Could you check a few things on this model? Use its own coordinates, in mm. A direction names the side the tool comes from. Round coordinates to 2 decimals unless told otherwise and drop trailing zeros. Loops run counter-clockwise (first coordinate to the right, second up) from the corner with the lowest first, then second, coordinate; pieces in that order, holes last. Notation, with made-up numbers: (-34.5, -8) - (23.5, -8) arc R22 ccw to (23.5, 28) - close; hole circle Ø1 at (-26.5, -32). An arc over 180 degrees is marked (long way). Answer as CSV lines item,"result". Start each with the question number.
1) Suppose I cut it at B-B, the plane z = 96. Count the separate pieces of the cut face and the enclosed holes in it, then the cut area to 3 significant figures.
2) I'm going to push flat-ended pins straight in: pin 1 Ø3.5 at (y, z) = (0.5, 80.5) entering from +X; pin 2 Ø5 at (x, y) = (16, 1.5) entering from +Z; pin 3 Ø0.5 at (x, z) = (29.5, 173.5) entering from -Y; pin 4 Ø0.5 at (x, z) = (29, 80) entering from +Y. Where does each tip first touch, or does it pass through?
3) Please list where these lines run through material, in increasing order: line 1 along X through (y, z) = (8, 193); line 2 along X through (y, z) = (-1, 208); line 3 along Y through (x, z) = (8, 213).
4) We'd pull the mould along Y, two halves only. Please class faces 5 (the face through (-5, -10, 118)), 6 (the face through (-3.9, 0, 118)), 7 (the face through (23.9, 0, 118)), 8 (the face through (5, 5, 0)): pulls with the +Y half, pulls with the -Y half, needs draft (parallel to the pull), parting line crosses it, or undercut.
5) Suppose I cut it at A-A, the plane x = 10. Write out the boundary of the cut face in (y, z), then the cut area to 3 significant figures.
6) Which directions (+Z, -Z, +X, -X, +Y, -Y) give clear straight access to the entire face, cutting with the end or side of a thin tool? Please do faces 1 (the face through (10, 8.2, 118)), 2 (the face through (20, 3.9, 118)), 3 (the face through (5, 5, 240)), 4 (the face through (0, -3.9, 118)).
```python
from build123d import *

# Parameters (mm, degrees)
SALIENTE_EXTRUIR1_DEPTH = 240


with BuildPart() as part:
    # Croquis1 → Saliente-Extruir1 (new body)
    with BuildSketch(Plane.XY):
        with BuildLine():
            Line((-10, 8.5), (-10, 2.3))
            Line((-10, 2.3), (-8.2, 2.3))
            Line((-8.2, 2.3), (-8.2, 5.5))
            Line((-8.2, 5.5), (-6.348528137, 5.5))
            Line((-6.348528137, 5.5), (-4.485786438, 3.6372583))
            ThreePointArc((-4.485786438, 3.6372583), (-4.052240935, 2.988411603), (-3.9, 2.223044738))
            Line((-3.9, 2.223044738), (-3.9, 0))
            Line((-3.9, 0), (-3.9, -2.223044738))
            ThreePointArc((-3.9, -2.223044738), (-4.052240935, -2.988411603), (-4.485786438, -3.6372583))
            Line((-4.485786438, -3.6372583), (-6.348528137, -5.5))
            Line((-6.348528137, -5.5), (-8.2, -5.5))
            Line((-8.2, -5.5), (-8.2, -2.3))
            Line((-8.2, -2.3), (-10, -2.3))
            Line((-10, -2.3), (-10, -8.5))
            ThreePointArc((-10, -8.5), (-9.560660172, -9.560660172), (-8.5, -10))
            Line((-8.5, -10), (-2.3, -10))
            Line((-2.3, -10), (-2.3, -8.2))
            Line((-2.3, -8.2), (-5.5, -8.2))
            Line((-5.5, -8.2), (-5.5, -6.348528137))
            Line((-5.5, -6.348528137), (-3.6372583, -4.485786438))
            ThreePointArc((-3.6372583, -4.485786438), (-2.988411603, -4.052240935), (-2.223044738, -3.9))
            Line((-2.223044738, -3.9), (0, -3.9))
            Line((0, -3.9), (2.223044738, -3.9))
            ThreePointArc((2.223044738, -3.9), (2.988411603, -4.052240935), (3.6372583, -4.485786438))
            Line((3.6372583, -4.485786438), (5.5, -6.348528137))
            Line((5.5, -6.348528137), (5.5, -8.2))
            Line((5.5, -8.2), (2.3, -8.2))
            Line((2.3, -8.2), (2.3, -10))
            Line((2.3, -10), (17.7, -10))
            Line((17.7, -10), (17.7, -8.2))
            Line((17.7, -8.2), (14.5, -8.2))
            Line((14.5, -8.2), (14.5, -6.348528137))
            Line((14.5, -6.348528137), (16.3627417, -4.485786438))
            ThreePointArc((16.3627417, -4.485786438), (17.011588397, -4.052240935), (17.776955262, -3.9))
            Line((17.776955262, -3.9), (20, -3.9))
            Line((20, -3.9), (22.223044738, -3.9))
            ThreePointArc((22.223044738, -3.9), (22.988411603, -4.052240935), (23.6372583, -4.485786438))
            Line((23.6372583, -4.485786438), (25.5, -6.348528137))
            Line((25.5, -6.348528137), (25.5, -8.2))
            Line((25.5, -8.2), (22.3, -8.2))
            Line((22.3, -8.2), (22.3, -10))
            Line((22.3, -10), (28.5, -10))
            ThreePointArc((28.5, -10), (29.560660172, -9.560660172), (30, -8.5))
            Line((30, -8.5), (30, -2.3))
            Line((30, -2.3), (28.2, -2.3))
            Line((28.2, -2.3), (28.2, -5.5))
            Line((28.2, -5.5), (26.348528137, -5.5))
            Line((26.348528137, -5.5), (24.485786438, -3.6372583))
            ThreePointArc((24.485786438, -3.6372583), (24.052240935, -2.988411603), (23.9, -2.223044738))
            Line((23.9, -2.223044738), (23.9, 0))
            Line((23.9, 0), (23.9, 2.223044738))
            ThreePointArc((23.9, 2.223044738), (24.052240935, 2.988411603), (24.485786438, 3.6372583))
            Line((24.485786438, 3.6372583), (26.348528137, 5.5))
            Line((26.348528137, 5.5), (28.2, 5.5))
            Line((28.2, 5.5), (28.2, 2.3))
            Line((28.2, 2.3), (30, 2.3))
            Line((30, 2.3), (30, 8.5))
            ThreePointArc((30, 8.5), (29.560660172, 9.560660172), (28.5, 10))
            Line((28.5, 10), (22.3, 10))
            Line((22.3, 10), (22.3, 8.2))
            Line((22.3, 8.2), (25.5, 8.2))
            Line((25.5, 8.2), (25.5, 6.348528137))
            Line((25.5, 6.348528137), (23.6372583, 4.485786438))
            ThreePointArc((23.6372583, 4.485786438), (22.988411603, 4.052240935), (22.223044738, 3.9))
            Line((22.223044738, 3.9), (20, 3.9))
            Line((20, 3.9), (17.776955262, 3.9))
            ThreePointArc((17.776955262, 3.9), (17.011588397, 4.052240935), (16.3627417, 4.485786438))
            Line((16.3627417, 4.485786438), (14.5, 6.348528137))
            Line((14.5, 6.348528137), (14.5, 8.2))
            Line((14.5, 8.2), (17.7, 8.2))
            Line((17.7, 8.2), (17.7, 10))
            Line((17.7, 10), (2.3, 10))
            Line((2.3, 10), (2.3, 8.2))
            Line((2.3, 8.2), (5.5, 8.2))
            Line((5.5, 8.2), (5.5, 6.348528137))
            Line((5.5, 6.348528137), (3.6372583, 4.485786438))
            ThreePointArc((3.6372583, 4.485786438), (2.988411603, 4.052240935), (2.223044738, 3.9))
            Line((2.223044738, 3.9), (0, 3.9))
            Line((0, 3.9), (-2.223044738, 3.9))
            ThreePointArc((-2.223044738, 3.9), (-2.988411603, 4.052240935), (-3.6372583, 4.485786438))
            Line((-3.6372583, 4.485786438), (-5.5, 6.348528137))
            Line((-5.5, 6.348528137), (-5.5, 8.2))
            Line((-5.5, 8.2), (-2.3, 8.2))
            Line((-2.3, 8.2), (-2.3, 10))
            Line((-2.3, 10), (-8.5, 10))
            ThreePointArc((-8.5, 10), (-9.560660172, 9.560660172), (-10, 8.5))
        make_face()
        with BuildLine():
            Line((3.9, 2.223044738), (3.9, 0))
            Line((3.9, 0), (3.9, -2.223044738))
            ThreePointArc((3.9, -2.223044738), (4.052240935, -2.988411603), (4.485786438, -3.6372583))
            Line((4.485786438, -3.6372583), (6.333883476, -5.485355339))
            ThreePointArc((6.333883476, -5.485355339), (6.604849416, -5.890884525), (6.7, -6.369238816))
            Line((6.7, -6.369238816), (6.7, -8.2))
            Line((6.7, -8.2), (13.3, -8.2))
            Line((13.3, -8.2), (13.3, -6.369238816))
            ThreePointArc((13.3, -6.369238816), (13.395150584, -5.890884525), (13.666116524, -5.485355339))
            Line((13.666116524, -5.485355339), (15.514213562, -3.6372583))
            ThreePointArc((15.514213562, -3.6372583), (15.947759065, -2.988411603), (16.1, -2.223044738))
            Line((16.1, -2.223044738), (16.1, 0))
            Line((16.1, 0), (16.1, 2.223044738))
            ThreePointArc((16.1, 2.223044738), (15.947759065, 2.988411603), (15.514213562, 3.6372583))
            Line((15.514213562, 3.6372583), (13.666116524, 5.485355339))
            ThreePointArc((13.666116524, 5.485355339), (13.395150584, 5.890884525), (13.3, 6.369238816))
            Line((13.3, 6.369238816), (13.3, 8.2))
            Line((13.3, 8.2), (6.7, 8.2))
            Line((6.7, 8.2), (6.7, 6.369238816))
            ThreePointArc((6.7, 6.369238816), (6.604849416, 5.890884525), (6.333883476, 5.485355339))
            Line((6.333883476, 5.485355339), (4.485786438, 3.6372583))
            ThreePointArc((4.485786438, 3.6372583), (4.052240935, 2.988411603), (3.9, 2.223044738))
        make_face(mode=Mode.SUBTRACT)
        with BuildLine():
            ThreePointArc((0, 2.5), (-1.767766953, 1.767766953), (-2.5, 0))
            ThreePointArc((-2.5, 0), (-1.767766953, -1.767766953), (0, -2.5))
            ThreePointArc((0, -2.5), (1.767766953, -1.767766953), (2.5, 0))
            ThreePointArc((2.5, 0), (1.767766953, 1.767766953), (0, 2.5))
        make_face(mode=Mode.SUBTRACT)
        with BuildLine():
            ThreePointArc((20, 2.5), (18.232233047, 1.767766953), (17.5, 0))
            ThreePointArc((17.5, 0), (18.232233047, -1.767766953), (20, -2.5))
            ThreePointArc((20, -2.5), (21.767766953, -1.767766953), (22.5, 0))
            ThreePointArc((22.5, 0), (21.767766953, 1.767766953), (20, 2.5))
        make_face(mode=Mode.SUBTRACT)
    extrude(amount=SALIENTE_EXTRUIR1_DEPTH)


solid = part.part
```
Filled sheet:
1,separate pieces,"1"
1,enclosed holes,"3"
1,area,"304 mm²"
2,pin 1,"x = 23.9"
2,pin 2,"z = 240"
2,pin 3,"y = -9.8"
2,pin 4,"y = 9.98"
3,line 1,"-10 to -5.5, 5.5 to 6.7, 13.3 to 14.5, 25.5 to 30"
3,line 2,"-3.9 to -2.29, 2.29 to 3.9, 16.1 to 17.71, 22.29 to 23.9"
3,line 3,"-10 to -8.2, 8.2 to 10"
4,face 5,"pulls with the -Y half"
4,face 6,"undercut"
4,face 7,"undercut"
4,face 8,"needs draft"
5,outline,"(-10, 0) - (-8.2, 0) - (-8.2, 240) - (-10, 240) - close; (8.2, 0) - (10, 0) - (10, 240) - (8.2, 240) - close"
5,area,"864 mm²"
6,face 1,"+Z, -Z"
6,face 2,"+Z, -Z, +Y"
6,face 3,"+Z, +X, -X, +Y, -Y"
6,face 4,"+Z, -Z, -Y"
